Source: CAD feature listing. Evaluate the final solid. Frame: model axes, mm. A direction names the side the tool comes from. Coordinates: 2 decimals unless noted, no trailing zeros. Write each loop counter-clockwise with the first axis right and the second up, starting at its lowest first coordinate (ties: lowest second). Pieces come first, ordered by that corner, then holes. Notation, with made-up numbers: M 78,71 L 100,71 A19 ccw 100,78 Z; hole C 67,70.5 d10. An arc over 180 degrees is marked long. Answer as CSV lines item,"result". Start each with the question number.
1. Reachability of faces 4 (the face through (0, -18, 41)), 5 (the face through (41, 0, 15)), 6 (the face through (-44, -25, 7)), 7 (the face through (44, -25, 7)), 8 (the face through (44, 25, 7)) from +Z, -Z, +X, -X, +Y, -Y: full face, straight path, thin tool, end or side. Return the list, or none.
2. Section C-C on z = 11. Return the cut outline in (x, y), plus the area to 3 significant figures.
3. Contact query for flat-ended pins moving along their axis: pin 1 Ø17.5 at (x, y) = (3.5, -5.5) entering from +Z; pin 2 Ø4.5 at (x, z) = (-46, 4.5) entering from -Y; pin 3 Ø7.5 at (x, z) = (-44, 6.5) entering from +Y; pin 4 Ø15 at (x, y) = (-55, 0) entering from -Z. Output: stop coordinate, or through.
4. Section A-A on y = 0. Return the cut outline in (x, z), plus the area to 3 significant figures.
5. Section D-D on y = 15. Return the cut outline in (x, z).
6. Line query: probe 1 along X at (y, z) = (0, 3.75); probe 2 along Y at (x, z) = (55, 7); probe 3 along Z at (x, y) = (34.5, -1.5). Output: solid intervals per line, ascending. Write a range as [from, to].
7. Section B-B on z = 34. Return the cut outline in (x, y).
8. Mould query, pull axis Y, two halves, no side actions, for faces 1 (the face through (-17.563, -0.56, 29.58)), 2 (the face through (0, 40, 24)), 3 (the face through (0, 18, 41)). Classes: pulls with the +Y half, pulls with the -Y half, needs draft (parallel to the pull), parting line crosses it, or undercut.
```python
from build123d import *

# Parameters (mm, degrees)
F0_R      = 12.5
F1_DEPTH  = 60
F2_W      = 25
F2_H      = 45
F3_DEPTH  = 80
F4_DEPTH  = 15
F6_DEPTH  = 15
F7_W      = 36
F7_H      = 30
F8_DEPTH  = 50
F8_FACE_W = 36
F8_FACE_H = 30
F9_DEPTH  = 25


with BuildPart() as f1:
    # F0 (on Top) → F1 (new body)
    with BuildSketch(Plane.XY):
        with BuildLine():
            Line((-55, -25), (55, -25))
            ThreePointArc((55, -25), (80, 0), (55, 25))
            Line((55, 25), (-55, 25))
            ThreePointArc((-55, 25), (-80, 0), (-55, -25))
        make_face()
        with Locations((-55, 0)):
            Circle(F0_R, mode=Mode.SUBTRACT)
        with Locations((55, 0)):
            Circle(F0_R, mode=Mode.SUBTRACT)
    extrude(amount=F1_DEPTH)

    # F2 (on face) → F3 (cut)
    with BuildSketch(Plane.XZ.offset(25)):
        with Locations((-67.5, 37.5)):
            Rectangle(F2_W, F2_H)
        Polygon((0, 60), (-55, 60), (-55, 15), (-25.980762, 15), align=None)
        Polygon((55, 60), (0, 60), (25.980762, 15), (55, 15), align=None)
        with Locations((67.5, 37.5)):
            Rectangle(F2_W, F2_H)
    extrude(amount=-F3_DEPTH, mode=Mode.SUBTRACT)

    # F2 (on face) → F4 (join)
    with BuildSketch(Plane.XZ.offset(25)):
        Polygon((25.980762, 15), (0, 60), (-25.980762, 15), (-34.641016, 0), (0, 0), (34.641016, 0), align=None)
    extrude(amount=F4_DEPTH)

    # F5 (on face) → F6 (join)
    with BuildSketch(Plane(origin=(0, 25, 0), x_dir=(-1, 0, 0), z_dir=(0, 1, 0))):
        Polygon((25.980762, 15), (0, 60), (-25.980762, 15), (-34.641016, 0), (34.641016, 0), align=None)
    extrude(amount=F6_DEPTH)

    # F7 (on Right) → F8 (cut)
    with BuildSketch(Plane.YZ):
        with Locations((0, 45)):
            Rectangle(F7_W, F7_H)
    extrude(amount=F8_DEPTH, mode=Mode.SUBTRACT)

    # F8_face (on face) → F9 (cut)
    with BuildSketch(Plane(origin=(0, 0, 45), x_dir=(0, 1, 0), z_dir=(1, 0, 0))):
        Rectangle(F8_FACE_W, F8_FACE_H)
    extrude(amount=-F9_DEPTH, mode=Mode.SUBTRACT)


solid = f1.part
```
Values:
1,face 4,"+Z, +X, -X"
1,face 5,"+Z, +X, +Y, -Y"
1,face 6,"+Z, -X, -Y"
1,face 7,"+Z, +X, -Y"
1,face 8,"+Z, +X, +Y"
2,outline,"M -55,-25 L -28.29,-25 L -28.29,-40 L 28.29,-40 L 28.29,-25 L 55,-25 A25 ccw 55,25 L 28.29,25 L 28.29,40 L -28.29,40 L -28.29,25 L -55,25 A25 ccw Z; hole C -55,0 d25; hole C 55,0 d25"
2,area,"8,180 mm²"
3,pin 1,"z = 30"
3,pin 2,"y = -25"
3,pin 3,"y = 25"
3,pin 4,"through"
4,outline,"M -80,0 L -67.5,0 L -67.5,15 L -80,15 Z; M -42.5,0 L 42.5,0 L 42.5,15 L 25.98,15 L 17.32,30 L -17.32,30 L -25.98,15 L -42.5,15 Z; M 67.5,0 L 80,0 L 80,15 L 67.5,15 Z"
4,area,"2,300 mm²"
5,outline,"M -75,0 L 75,0 L 75,15 L 25.98,15 L 17.32,30 L -17.32,30 L -25.98,15 L -75,15 Z"
6,probe 1,"[-80, -67.5], [-42.5, 42.5], [67.5, 80]"
6,probe 2,"[-25, -12.5], [12.5, 25]"
6,probe 3,"[0, 15]"
7,outline,"M -15.01,-40 L 15.01,-40 L 15.01,-18 L -15.01,-18 Z; M -15.01,18 L 15.01,18 L 15.01,40 L -15.01,40 Z"
8,face 1,"needs draft"
8,face 2,"pulls with the +Y half"
8,face 3,"undercut"
